Geometry check sheet. Reference: drawing and pictorial views, mm from the part's lowest x, y, z. Give positions to 0.01 mm unless a question says otherwise; leave off trailing zeros. Write each loop counter-clockwise with the first axis right and the second up, starting at its lowest first coordinate (ties: lowest second). Pieces come first, ordered by that corner, then holes. Notation, with made-up numbers: (-2.75, 22) -> (26.25, 22) arc R32 ccw to (26.25, 54) -> close; hole circle Ø4 at (-11.5, -22.5). An arc over 180 degrees is marked (long way). Return JSON: item names as keys, results as strings.
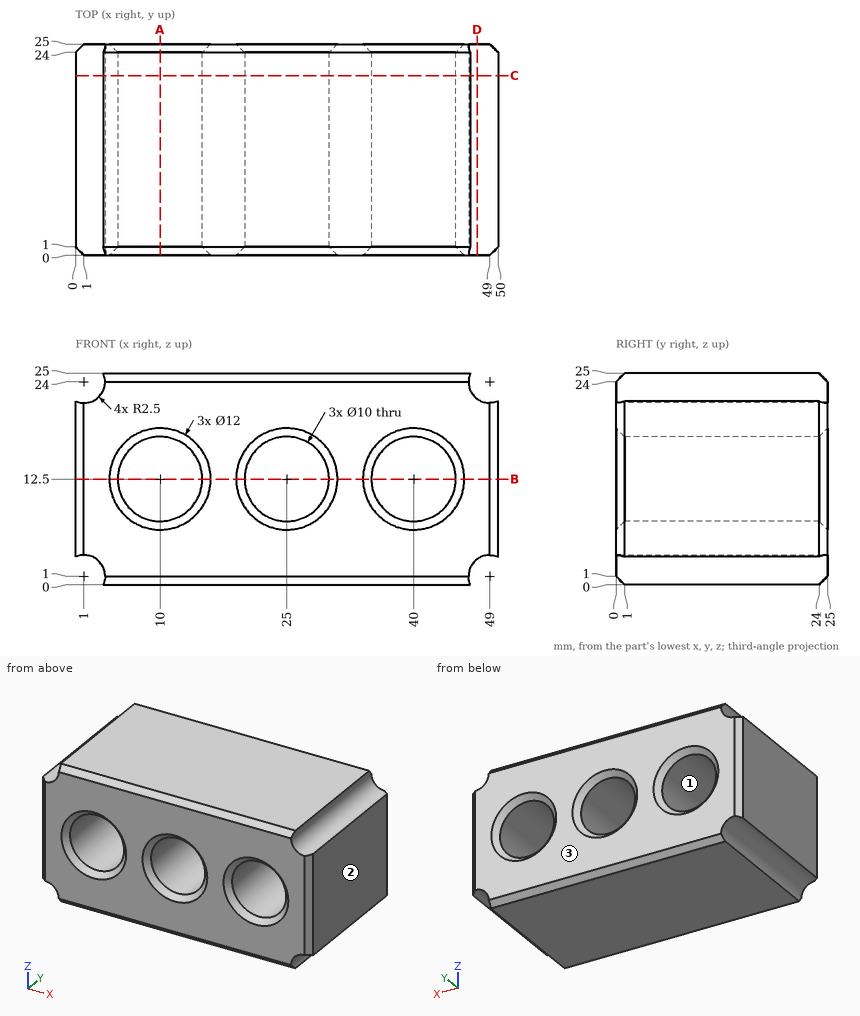
(1) Cross-section at D-D on x = 47.5. Enter the section's corners in (y, z), then the cut area to 3 significant figures.
Reply:
{"outline": "(0, 3) -> (25, 3) -> (25, 22) -> (0, 22) -> close", "area": "475 mm^2"}
(2) Cross-section at C-C on y = 21.25. Enter the section's corners in (x, z), then the cut area to 3 significant figures.
Reply:
{"outline": "(0, 3.29) arc R2.5 cw to (3.29, 0) -> (46.71, 0) arc R2.5 cw to (50, 3.29) -> (50, 21.71) arc R2.5 cw to (46.71, 25) -> (3.29, 25) arc R2.5 cw to (0, 21.71) -> close; hole circle Ø10 at (10, 12.5); hole circle Ø10 at (25, 12.5); hole circle Ø10 at (40, 12.5)", "area": "971 mm^2"}
(3) Cross-section at B-B on z = 12.5. State how many separate pieces and enclosed holes the cut face has, then the cut area to 3 significant figures.
Reply:
{"separate pieces": "4", "enclosed holes": "0", "area": "492 mm^2"}
(4) Thickness scan on L1, parallel to Z at x = 10, y = 14; L2, parallel to X at y = 2.25, z = 16.25; L3, parallel to X at y = 22.5, z = 8.5. Record the ranges inside material, lowest first.
Reply:
{"L1": "0 to 7.5, 17.5 to 25", "L2": "0 to 6.69, 13.31 to 21.69, 28.31 to 36.69, 43.31 to 50", "L3": "0 to 7, 13 to 22, 28 to 37, 43 to 50"}
(5) Depth check by flat-ended pin: pin 1 Ø11.5 at (x, z) = (10, 12.5) entering from +Y. Enter the tip coordinate at first touch or a pass-through.
Reply:
{"pin 1": "y = 24.75"}
(6) Release check for a two-part mould opening along X. For the marked faces 1, 2 and 3 record: pulls with the +X half, pulls with the -X half, needs draft (parallel to the pull), parting line crosses it, or undercut.
Reply:
{"face 1": "undercut", "face 2": "pulls with the +X half", "face 3": "needs draft"}
(7) Cross-section at A-A on x = 10. Enter the section's corners in (y, z), then the cut area to 3 significant figures.
Reply:
{"outline": "(0, 1) -> (1, 0) -> (24, 0) -> (25, 1) -> (25, 6.5) -> (24, 7.5) -> (1, 7.5) -> (0, 6.5) -> close; (0, 18.5) -> (1, 17.5) -> (24, 17.5) -> (25, 18.5) -> (25, 24) -> (24, 25) -> (1, 25) -> (0, 24) -> close", "area": "371 mm^2"}
